Source: three-view drawing plus pictorial views. Frame: mm from the lowest corner of the part. A direction names the side the tool comes from. Give positions to 0.01 mm unless a question says otherwise; leave off trailing zeros. Order: outer loops, then holes, each group sorted by start corner. A loop starts at its lowest first (then second) coordinate and runs counter-clockwise, first axis right, second up.
1) Section D-D, the plane x = 23. Return loops of the section in (y, z).
2) First-contact query: P1, Ø5, axis at x = 26, y = 9, coming from the -Z side; P2, Ø1, axis at y = 1, z = 6, coming from the -X side; P3, Ø0.6, axis at x = 26.5, z = 7.5, coming from the -Y side; P4, Ø1, axis at y = 4, z = 10.5, coming from the +X side. Flat tips, straight axial feed; report the tip coordinate or a pass-through.
3) Material intervals for line 1 (Y direction, x = 51, z = 10.75); line 2 (Z direction, x = 35.5, y = 11); line 3 (X direction, y = 8.25, z = 7.5) (1 decimal), sorted ascending.
4) Section A-A, the plane y = 5.25. Return loops of the section in (x, z) (1 decimal), plus the area to 3 significant figures.
5) Section B-B, the plane z = 2.5. Return loops of the section in (x, y) (1 decimal).
6) Access query for the marked faces 1 and 2. Directions: +Z, -Z, +X, -X, +Y, -Y. A direction counts if a zero-diameter tool reaches every point of the face in a straight line with its end or side. Return the directions, or none.
7) Section C-C, the plane y = 1.5. Give the number of separate pieces and of enclosed holes in the cut face, plus the area to 3 significant figures.
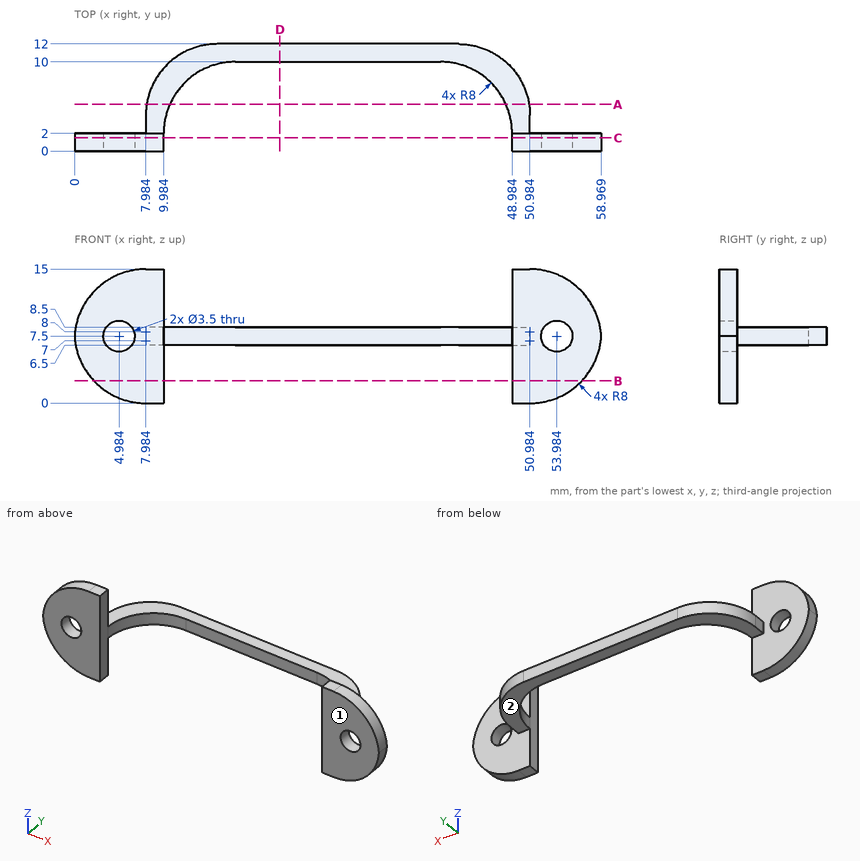
From the geometry:
1. outline: (10, 6.5) - (12, 6.5) - (12, 8.5) - (10, 8.5) - close
2. P1: stops at z = 6.5
2. P2: stops at x = 0.13
2. P3: stops at y = 10
2. P4: passes through
3. line 1: y = 0 to 2
3. line 2: z = 6.5 to 8.5
3. line 3: x = 9.2 to 13, 46 to 49.8
4. outline: (8.1, 6.5) - (10.7, 6.5) - (10.7, 8.5) - (8.1, 8.5) - close; (48.3, 6.5) - (50.9, 6.5) - (50.9, 8.5) - (48.3, 8.5) - close
4. area: 10.4 mm2
5. outline: (2.2, 0) - (10, 0) - (10, 2) - (2.2, 2) - close; (49, 0) - (56.8, 0) - (56.8, 2) - (49, 2) - close
6. face 1: +Z, -Z, +X, -X, -Y
6. face 2: -Z, +X, -X, +Y
7. separate pieces: 2
7. enclosed holes: 2
7. area: 226 mm2
